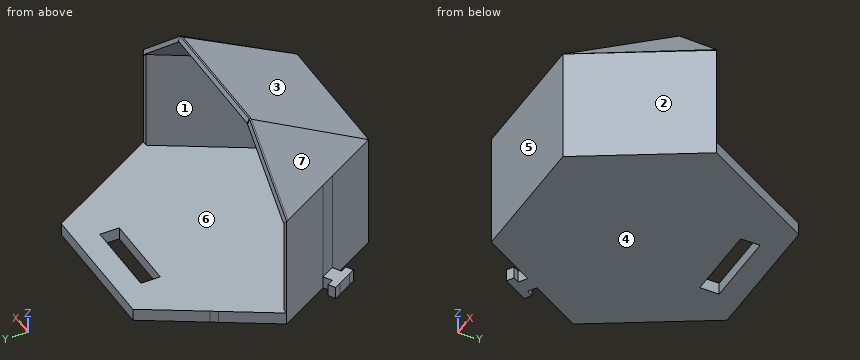
from build123d import *

# Parameters (mm, degrees)
F0_W      = 50
F0_H      = 12.5
F1_DEPTH  = 8
F2_DEPTH  = 75
F4_DEPTH  = 8
F7_DEPTH  = 3
F8_DEPTH  = 1
F11_DEPTH = 3
F14_DEPTH = 3
F15_DEPTH = 8
F16_DEPTH = 8
F17_DEPTH = 12.5


# Not quite as in the source:
# - a feature names something its author has since deleted; it is built from what else it names


with BuildPart() as f1:
    # F0 (on Top) → F1 (new body)
    with BuildSketch(Plane.XY):
        Polygon((42.0179491924, -72.7772228311), (84.0358983849, 0), (42.0179491924, 72.7772228311), (-42.0179491924, 72.7772228311), (-84.0358983849, 0), (-42.0179491924, -72.7772228311), align=None)
        with Locations((0, 54.5829171234)):
            Rectangle(F0_W, F0_H, mode=Mode.SUBTRACT)
    extrude(amount=F1_DEPTH)

    # F0 (on Top) → F2 (join)
    with BuildSketch(Plane.XY):
        Polygon((43.75, -75.7772228311), (87.5, 0), (84.0358983849, 0), (42.0179491924, -72.7772228311), (-42.0179491924, -72.7772228311), (-84.0358983849, 0), (-87.5, 0), (-68.1246734519, -33.5590499945), (-63.1805508476, -42.1225215441), (-43.75, -75.7772228311), align=None)
    extrude(amount=F2_DEPTH)

    # F0 (on Top) → F4 (join)
    with BuildSketch(Plane.XY):
        Polygon((43.75, 75.7772228311), (-43.75, 75.7772228311), (-65.625, 37.8886114156), (-68.125, 33.5584843966), (-87.5, 0), (-84.0358983849, 0), (-42.0179491924, 72.7772228311), (42.0179491924, 72.7772228311), (84.0358983849, 0), (87.5, 0), align=None)
    extrude(amount=F4_DEPTH)

    # F6 (on face) → F7 (join)
    with BuildSketch(Plane(origin=(0, -50.1312366318, 89.3836679776), x_dir=(1, 0, 0), z_dir=(0, 0.4891706574, -0.872188092))):
        Polygon((43.75, 29.4041920927), (0, 29.4041920927), (-43.75, 29.4041920927), (-42.01795, -57.4775522498), (42.01795, -57.4775522498), align=None)
    extrude(amount=F7_DEPTH)

    # F3 (on Front) → F8 (join)
    with BuildSketch(Plane.XZ):
        Polygon((-42.01795, 114.5), (0, 114.5), (42.01795, 114.5), (84.0359, 75), (87.5, 75), (42.01795, 117.5), (0, 117.5), (-42.01795, 117.5), (-87.5, 75), (-84.0359, 75), align=None)
    extrude(amount=F8_DEPTH)

    # F10 (on face) → F11 (join)
    with BuildSketch(Plane(origin=(-67.6846727043, -39.0777640058, 72.4338274863), x_dir=(0.7723629594, -0.3015876344, 0.5590173143), z_dir=(-0.6351814378, -0.3667221741, 0.6797495039))):
        Polygon((33.2314262259, 55.789645187), (-25.6554603702, 35.6104118215), (30.9888924807, -31.0804218073), align=None)
    extrude(amount=-F11_DEPTH)

    # F13 (on face) → F14 (join)
    with BuildSketch(Plane(origin=(67.6756688636, -39.5950852503, 72.4241918832), x_dir=(0.7733047167, 0.3041472681, -0.556322078), z_dir=(-0.6340345536, 0.3709553614, -0.6785221475))):
        Polygon((-30.939509805, 30.5117392321), (-32.8751652468, -56.3649154418), (25.9400068576, -35.9776056011), align=None)
    extrude(amount=F14_DEPTH)

    # F0 (on Top) → F15 (join)
    with BuildSketch(Plane.XY):
        with Locations((0, 54.5829171234)):
            Rectangle(F0_W, F0_H)
    extrude(amount=F15_DEPTH)

    # F0 (on Top) → F16 (join)
    with BuildSketch(Plane.XY):
        Polygon((-77.8456263738, -39.3203930924), (-73.5443197712, -36.7711262349), (-75.7943197712, -32.8740119179), (-80.0956263738, -35.4232787754), align=None)
        Polygon((-63.1805508476, -42.1225215441), (-68.1246734519, -33.5590499945), (-73.5443197712, -36.7711262349), (-77.8456263738, -39.3203930924), (-72.8440428469, -47.9797326875), (-68.5681614313, -45.3880463409), align=None)
        Polygon((-66.2356437193, -49.236339615), (-68.5681614313, -45.3880463409), (-72.8440428469, -47.9797326875), (-70.5115251349, -51.8280259616), align=None)
    extrude(amount=F16_DEPTH)

    # F0 (on Top) → F17 (cut, symmetric)
    with BuildSketch(Plane.XY):
        with Locations((0, 54.5829171234)):
            Rectangle(F0_W, F0_H)
    extrude(amount=F17_DEPTH, both=True, mode=Mode.SUBTRACT)


solid = f1.part
CAD build for the part. Positions are in the model's coordinates, mm. Face numbers are marked on the shaded views. A direction names the side the tool comes from. Give positions to 0.01 mm unless a question says otherwise; leave off trailing zeros. Write each loop counter-clockwise with the first axis right and the second up, starting at its lowest first coordinate (ties: lowest second). Pieces come first, ordered by that corner, then holes. Notation, with made-up numbers: M -30,13.5 L -17,13.5 A19 cw -17,32.5 Z; hole C 61,58.25 d10. An arc over 180 degrees is marked long. Put each result on its own line as item: value. Start each with the question number.
(1) Band-saw the part on C-C, the plane y = -8. Write the cut outline in (x, z), and give its area (3 significant figures).
(2) Probe L1, parallel to Z at x = -18.5, y = 62.5; L2, parallel to X at y = -39.5, z = 46; L3, parallel to X at y = -26.5, z = 28.5. List the from-to ranges inside material, lowest first.
(3) Band-saw the part on A-A, the plane x = 31. Write the cut outline in (y, z), and give its area (3 significant figures).
(4) Mould opens along X. For the marked faces 5, 6 and 7 say: +X half, -X half, draft (parallel to the pull), parting line (faces both ways), or undercut.
(5) Which spindle directions (+Z, -Z, +X, -X, +Y, -Y) get a long thin tool onto all of the face, cutting with end or side? Do the marked faces 1, 2, 3 and 4. Say none if no direction does.
(6) Band-saw the part on D-D, the plane y = 52. Write the cut outline in (x, z), and give its area (3 significant figures).
(7) Flat gauge pins, fed straight in: pin 1 Ø19.5 at (x, z) = (-14.5, 39.5) entering from +Y; pin 2 Ø6.5 at (y, z) = (54.5, 4) entering from -X; pin 3 Ø4 at (x, z) = (-85, 29.5) entering from +Y. Where does each tip first touch, or does it go through?
(8) Band-saw the part on B-B, the plane z = 53. Write the cut outline in (x, y), and give its area (3 significant figures).
Response values:
1. outline: M -82.88,0 L 82.88,0 L 82.88,75 L 83.16,75.23 L 42.41,113.31 L 42.2,113.01 L -42.2,113.01 L -82.88,75 Z; hole M -79.42,8 L 79.42,8 L 79.42,74.3 L 41.67,109.57 L -41.16,109.57 L -79.42,73.82 Z
1. area: 2,420 mm2
2. L1: z = 0 to 8
2. L2: x = -64.69 to -61.23, 61.23 to 64.69
2. L3: x = -72.2 to -68.74, 68.74 to 72.2
3. outline: M -75.78,0 L 75.78,0 L 75.78,8 L -72.78,8 L -72.78,73.24 L 1.47,114.88 L 0,117.5 L -1,117.5 L -1,116.94 L -75.78,75 Z
3. area: 1,670 mm2
4. face 5: draft
4. face 6: undercut
4. face 7: -X half
5. face 1: +Y
5. face 2: -Z, +X, -Y
5. face 3: +Z, -X, -Y
5. face 4: -Z, +X, -X, +Y, -Y
6. outline: M -57.48,0 L -25,0 L -25,8 L -57.48,8 Z; M 25,0 L 57.48,0 L 57.48,8 L 25,8 Z
6. area: 520 mm2
7. pin 1: stops at y = -72.78
7. pin 2: stops at x = -57.91
7. pin 3: stops at y = 0
8. outline: M -87.5,0 L -43.75,-75.78 L 43.75,-75.78 L 87.5,0 L 84.04,0 L 42.02,-72.78 L -42.02,-72.78 L -84.04,0 Z
8. area: 772 mm2
